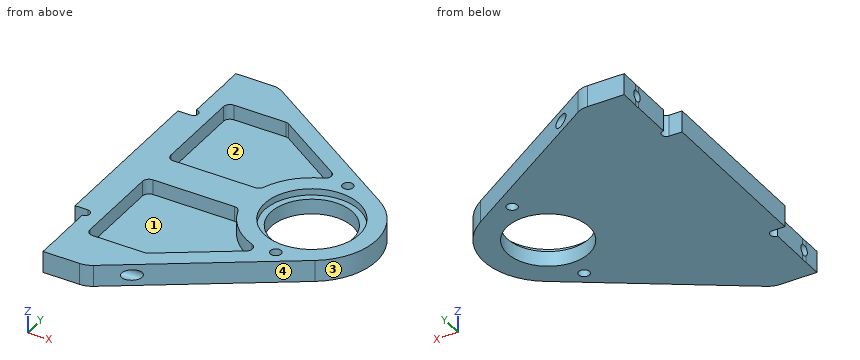
```python
from build123d import *

# Parameters (mm, degrees)
SKETCH_2_W          = 3
SKETCH_2_H          = 40
SKETCH_2_R          = 9.5
SKETCH_2_R_2        = 1.25
EXTRUDE_1_DEPTH     = 5
FILLET_3_R          = 5
SKETCH_3_R          = 1.25
CUT_EXTRUDE_1_DEPTH = 56
SKETCH_4_R          = 1.1
CUT_EXTRUDE_2_DEPTH = 10
SKETCH_5_R          = 2.1
CUT_EXTRUDE_3_DEPTH = 10
SKETCH_7_R          = 11
CUT_EXTRUDE_5_DEPTH = 1.5
CUT_EXTRUDE_6_DEPTH = 3.5
FILLET_5_R          = 1.5


with BuildPart() as part:
    # ｽｹｯﾁ2 → ﾎﾞｽ - 押し出し1 (new body)
    with BuildSketch(Plane.XY):
        with Locations((-41.5, 0)):
            Rectangle(SKETCH_2_W, SKETCH_2_H)
        with BuildLine():
            Line((-40, 37.5), (-40, -37.5))
            Line((-40, -37.5), (-30, -37.5))
            Line((-30, -37.5), (8.20017536, -12.560140288))
            ThreePointArc((8.20017536, -12.560140288), (15, 0), (8.20017536, 12.560140288))
            Line((8.20017536, 12.560140288), (-30, 37.5))
            Line((-30, 37.5), (-40, 37.5))
        make_face()
        Circle(SKETCH_2_R, mode=Mode.SUBTRACT)
        with Locations((0, 14)):
            Circle(SKETCH_2_R_2, mode=Mode.SUBTRACT)
        with Locations((0, -14)):
            Circle(SKETCH_2_R_2, mode=Mode.SUBTRACT)
    extrude(amount=EXTRUDE_1_DEPTH)

    # ﾌｨﾚｯﾄ3
    fillet_3_edges = [part.edges().sort_by_distance(p)[0] for p in [
        (-30, 37.5, 2.5),
        (-30, -37.5, 2.5),
    ]]
    fillet(fillet_3_edges, radius=FILLET_3_R)

    # ｽｹｯﾁ3 → ｶｯﾄ - 押し出し1 (cut, through all)
    with BuildSketch(Plane.ZY.offset(40)):
        with Locations((2.5, -32.5)):
            Circle(SKETCH_3_R)
        with Locations((2.5, 32.5)):
            Circle(SKETCH_3_R)
    extrude(amount=-CUT_EXTRUDE_1_DEPTH, mode=Mode.SUBTRACT)

    # ｽｹｯﾁ4 → ｶｯﾄ - 押し出し2 (cut)
    with BuildSketch(Plane(origin=(0, 0, 0), x_dir=(-1, 0, 0), z_dir=(0, 0, -1))):
        with Locations((40, 21.1)):
            Circle(SKETCH_4_R)
        with Locations((40, -21.1)):
            Circle(SKETCH_4_R)
    extrude(amount=-CUT_EXTRUDE_2_DEPTH, mode=Mode.SUBTRACT)

    # ｽｹｯﾁ5 → ｶｯﾄ - 押し出し3 (cut)
    with BuildSketch(Plane(origin=(0, 0, 0), x_dir=(-1, 0, 0), z_dir=(0, 0, -1))):
        with Locations((42, 32.5)):
            Circle(SKETCH_5_R)
        with Locations((42, -32.5)):
            Circle(SKETCH_5_R)
    extrude(amount=-CUT_EXTRUDE_3_DEPTH, mode=Mode.SUBTRACT)

    # ｽｹｯﾁ7 → ｶｯﾄ - 押し出し5 (cut)
    with BuildSketch(Plane.XY.offset(5)):
        Circle(SKETCH_7_R)
    extrude(amount=-CUT_EXTRUDE_5_DEPTH, mode=Mode.SUBTRACT)

    # ｽｹｯﾁ8 → ｶｯﾄ - 押し出し6 (cut)
    with BuildSketch(Plane.XY.offset(5)):
        with BuildLine():
            Line((-36, -4), (-36, -27.5))
            Line((-36, -27.5), (-22, -27.5))
            Line((-22, -27.5), (-2.525791459, -14.785816768))
            ThreePointArc((-2.525791459, -14.785816768), (-10.059117169, -11.127181214), (-14.456832295, -4))
            Line((-14.456832295, -4), (-36, -4))
        make_face()
        with BuildLine():
            Line((-22, 27.5), (-2.525791459, 14.785816768))
            ThreePointArc((-2.525791459, 14.785816768), (-10.059117169, 11.127181214), (-14.456832295, 4))
            Line((-14.456832295, 4), (-36, 4))
            Line((-36, 4), (-36, 27.5))
            Line((-36, 27.5), (-22, 27.5))
        make_face()
    extrude(amount=-CUT_EXTRUDE_6_DEPTH, mode=Mode.SUBTRACT)

    # ﾌｨﾚｯﾄ5
    fillet_5_edges = [part.edges().sort_by_distance(p)[0] for p in [
        (-36, 27.5, 3.25),
        (-22, 27.5, 3.25),
        (-2.525791459, 14.785816768, 3.25),
        (-14.456832295, 4, 3.25),
        (-36, 4, 3.25),
        (-22, -27.5, 3.25),
        (-36, -27.5, 3.25),
        (-36, -4, 3.25),
        (-14.456832295, -4, 3.25),
        (-2.525791459, -14.785816768, 3.25),
    ]]
    fillet(fillet_5_edges, radius=FILLET_5_R)


solid = part.part
```
Input: part model. Units: mm. Frame: model coordinates. Face numbers are marked on the shaded views. Give positions to 0.01 mm unless a question says otherwise; leave off trailing zeros. Loops run counter-clockwise (first coordinate to the right, second up) from the corner with the lowest first, then second, coordinate; pieces in that order, holes last. Notation, with made-up numbers: (55.5, 86) -> (84.5, 86) arc R22 ccw to (84.5, 123) -> close; hole circle Ø6 at (-31, 49.5). An arc over 180 degrees is marked (long way). Use a Markdown table: item, result.
Q1. First-contact query: P1, Ø1.5, axis at x = 0, y = -14, coming from the +Z side; P2, Ø3, axis at y = 32.5, z = 2.5, coming from the -X side; P3, Ø1, axis at x = -21, z = 4, coming from the -Y side; P4, Ø3, axis at y = 17, z = 4, coming from the +X side. Flat tips, straight axial feed; report the tip coordinate or a pass-through.
Entries:
| item | result |
|---|---|
| P1 | passes through |
| P2 | stops at x = -40 |
| P3 | stops at y = -31.95 |
| P4 | stops at x = 3.7 |
Q2. Section query C-C, the plane y = -21.1. Return the cut outline in (x, z), plus the area to 3 significant figures.
Entries:
| item | result |
|---|---|
| outline | (-38.9, 0) -> (-4.88, 0) -> (-4.88, 5) -> (-12.2, 5) -> (-12.2, 1.5) -> (-36, 1.5) -> (-36, 5) -> (-38.9, 5) -> close |
| area | 86.8 mm² |
Q3. Ray query, probe 1 along Y at (x, z) = (0, 4.55); probe 2 along Y at (x, z) = (-32, 2.7); probe 3 along Y at (x, z) = (0, 2.75). Return the intervals inside material, ascending. Write a range as from..to.
Entries:
| item | result |
|---|---|
| probe 1 | y = -17.91..-15.25, -12.75..-11, 11..12.75, 15.25..17.91 |
| probe 2 | y = -37.5..-33.73, -31.27..-27.5, -4..4, 27.5..31.27, 33.73..37.5 |
| probe 3 | y = -17.91..-15.25, -12.75..-9.5, 9.5..12.75, 15.25..17.91 |
Q4. Pull-direction query (Y, two-part tool) for the marked faces 1, 2, 3 and 4; classes: pulls with the +Y half, pulls with the -Y half, needs draft (parallel to the pull), parting line crosses it, or undercut.
Entries:
| item | result |
|---|---|
| face 1 | undercut |
| face 2 | undercut |
| face 3 | parting line crosses it |
| face 4 | pulls with the -Y half |
Q5. Section query B-B, the plane x = 0. Return the cut outline in (y, z), plus the area to 3 significant figures.
Entries:
| item | result |
|---|---|
| outline | (-17.91, 0) -> (-15.25, 0) -> (-15.25, 5) -> (-17.91, 5) -> close; (-12.75, 0) -> (-9.5, 0) -> (-9.5, 3.5) -> (-11, 3.5) -> (-11, 5) -> (-12.75, 5) -> close; (9.5, 0) -> (12.75, 0) -> (12.75, 5) -> (11, 5) -> (11, 3.5) -> (9.5, 3.5) -> close; (15.25, 0) -> (17.91, 0) -> (17.91, 5) -> (15.25, 5) -> close |
| area | 54.6 mm² |
Q6. Section query D-D, the plane z = 2.5. State how many separate pieces and enclosed holes the cut face has, plus the area to 3 significant figures.
Entries:
| item | result |
|---|---|
| separate pieces | 3 |
| enclosed holes | 5 |
| area | 1,380 mm² |
Q7. Section query A-A, the plane y = 0. Return the cut outline in (x, z).
Entries:
| item | result |
|---|---|
| outline | (-43, 0) -> (-9.5, 0) -> (-9.5, 3.5) -> (-11, 3.5) -> (-11, 5) -> (-43, 5) -> close; (9.5, 0) -> (15, 0) -> (15, 5) -> (11, 5) -> (11, 3.5) -> (9.5, 3.5) -> close |
